Can you work these out from the model? Positions are in its coordinate system, mm. A direction names the side the tool comes from. Give positions to 0.01 mm unless a question says otherwise; leave off trailing zeros. Order: outer loops, then holes, each group sorted by start corner. A loop starts at its lowest first (then second) coordinate and runs counter-clockwise, first axis right, second up. Notation, with made-up numbers: M 32,-19.75 L 42,-19.75 A12 ccw 42,3.25 Z; hole C -17,-40 d9. An arc over 180 degrees is marked long. Answer as a JSON object with one key per item and string values.
```python
from build123d import *

# Parameters (mm, degrees)
CBORE_START                                   = 1.6
CBORE_FOR_M3_HEX_SOCKET_HEAD_CAP_SCR_2_R      = 3.25
CBORE_FOR_M3_HEX_SOCKET_HEAD_CAP_SCREW1_DEPTH = 6.092474541
CBORE_FOR_M3_HEX_SOCKET_HEAD_CAP_SCR_3_O_R    = 1.7
CBORE_FOR_M3_HEX_SOCKET_HEAD_CAP_SCR_3_DEPTH  = 1.6


with BuildPart() as part:
    # Sketch1 → Revolve1 (revolve)
    with BuildSketch(Plane.XY, mode=Mode.PRIVATE) as revolve1_sk:
        with BuildLine():
            Line((0, 0), (17.5, 0))
            Line((17.5, 0), (17.5, 5))
            ThreePointArc((17.5, 5), (8.661165235, 8.661165235), (5, 17.5))
            Line((5, 17.5), (5, 91.339745962))
            Line((5, 91.339745962), (0, 100))
            Line((0, 100), (0, 0))
        make_face()
    revolve(revolve1_sk.sketch.rotate(Axis((0, 0, 0), (0, 1, 0)), 90), axis=Axis((0, 0, 0), (0, 1, 0)))

    # CBORE for M3 Hex Socket Head Cap Screw1: read off the stored shape, not the designer's step
    # CBORE for M3 Hex Socket Head Cap Scr 2 → CBORE for M3 Hex Socket Head Cap Screw1 (cut)
    with BuildSketch(Plane(origin=(0, 0, 0), x_dir=(1, 0, 0), z_dir=(0, 1, 0)).offset(CBORE_START)):
        with Locations((-6.5, -11.258330249)):
            Circle(CBORE_FOR_M3_HEX_SOCKET_HEAD_CAP_SCR_2_R)
        with Locations((6.5, -11.258330249)):
            Circle(CBORE_FOR_M3_HEX_SOCKET_HEAD_CAP_SCR_2_R)
        with Locations((13, 0)):
            Circle(CBORE_FOR_M3_HEX_SOCKET_HEAD_CAP_SCR_2_R)
        with Locations((6.5, 11.258330249)):
            Circle(CBORE_FOR_M3_HEX_SOCKET_HEAD_CAP_SCR_2_R)
        with Locations((-6.5, 11.258330249)):
            Circle(CBORE_FOR_M3_HEX_SOCKET_HEAD_CAP_SCR_2_R)
        with Locations((-13, 0)):
            Circle(CBORE_FOR_M3_HEX_SOCKET_HEAD_CAP_SCR_2_R)
    extrude(amount=CBORE_FOR_M3_HEX_SOCKET_HEAD_CAP_SCREW1_DEPTH, mode=Mode.SUBTRACT)

    # CBORE for M3 Hex Socket Head Cap Scr 3 o → CBORE for M3 Hex Socket Head Cap Scr 3 (cut)
    with BuildSketch(Plane(origin=(0, 0, 0), x_dir=(1, 0, 0), z_dir=(0, 1, 0))):
        with Locations((-6.5, -11.258330249)):
            Circle(CBORE_FOR_M3_HEX_SOCKET_HEAD_CAP_SCR_3_O_R)
        with Locations((6.5, -11.258330249)):
            Circle(CBORE_FOR_M3_HEX_SOCKET_HEAD_CAP_SCR_3_O_R)
        with Locations((13, 0)):
            Circle(CBORE_FOR_M3_HEX_SOCKET_HEAD_CAP_SCR_3_O_R)
        with Locations((6.5, 11.258330249)):
            Circle(CBORE_FOR_M3_HEX_SOCKET_HEAD_CAP_SCR_3_O_R)
        with Locations((-6.5, 11.258330249)):
            Circle(CBORE_FOR_M3_HEX_SOCKET_HEAD_CAP_SCR_3_O_R)
        with Locations((-13, 0)):
            Circle(CBORE_FOR_M3_HEX_SOCKET_HEAD_CAP_SCR_3_O_R)
    extrude(amount=CBORE_FOR_M3_HEX_SOCKET_HEAD_CAP_SCR_3_DEPTH, mode=Mode.SUBTRACT)


solid = part.part
```
1) I want a section at B-B on x = 6.5. Count the separate pieces of the cut face and the enclosed holes in it, and give its area (3 significant figures).
Results found:
{"separate pieces": "3", "enclosed holes": "0", "area": "183 mm²"}
2) I'm going to push flat-ended pins straight in: pin 1 Ø1.5 at (x, y) = (-2, 70) entering from -Z; pin 2 Ø4 at (x, z) = (-4.5, -7) entering from -Y; pin 3 Ø7 at (x, z) = (8, -10) entering from +Y; pin 4 Ø7 at (x, z) = (5.5, 10) entering from +Y. Where does each tip first touch, or does it pass through?
Results found:
{"pin 1": "stops at z = -4.84", "pin 2": "stops at y = 0", "pin 3": "stops at y = 8.06", "pin 4": "stops at y = 9.48"}
3) I need wall thicknesses on L1, parallel to X at y = 4.25, z = 0; L2, parallel to X at y = 0.4, z = 0; L3, parallel to Z at x = -6.5, y = 1.25. Which ranges of each line are inside material? Lowest first, please.
Results found:
{"L1": "x = -17.5 to -16.25, -9.75 to 9.75, 16.25 to 17.5", "L2": "x = -17.5 to -14.7, -11.3 to 11.3, 14.7 to 17.5", "L3": "z = -16.25 to -12.96, -9.56 to 9.56, 12.96 to 16.25"}
4) I want a section at A-A on y = 24. Write out the boundary of the cut face in (x, z), and give its area (3 significant figures).
Results found:
{"outline": "C 0,0 d10", "area": "78.5 mm²"}
5) Thinking about a two-plate mould opening in X: for faces 3 (the face through (0, 0, 0)), 4 (the face through (17.084, 2.535, 3.794)), 5 (the face through (-11.43, 0.79, 0.65)), 6 (the face through (14.4, 1.6, 1.4)), which applies, pulls with the +X half, pulls with the -X half, needs draft (parallel to the pull), parting line crosses it, or undercut?
Results found:
{"face 3": "needs draft", "face 4": "parting line crosses it", "face 5": "undercut", "face 6": "undercut"}
6) For faces 1 (the face through (-11.6, 1.6, 1.4)), 2 (the face through (-6.721, 0.789, -12.944)), which set-ups out of +Z, -Z, +X, -X, +Y, -Y let a thin tool reach every point of the face, with its end or its side?
Results found:
{"face 1": "+Y", "face 2": "+Y, -Y"}
